Verification items for the finished model (mm, model axes). Coordinates: 2 decimals unless noted, no trailing zeros. Order: outer loops, then holes, each group sorted by start corner. A loop starts at its lowest first (then second) coordinate and runs counter-clockwise, first axis right, second up. Notation, with made-up numbers: M -30,34 L 2,34 A31 ccw 2,68 Z; hole C 8,65 d7. An arc over 180 degrees is marked long. Answer as a JSON object with one key per item and string values. Group by question number.
(1) Cross-section at B-B (y = 38). Enter the section's corners in (x, z).
(2) Cross-section at C-C (x = 34). Enter the section's corners in (y, z).
(3) Gauge pin test, flat ends, axial feed: pin 1 Ø0.9 at (y, z) = (62, 2) entering from -X; pin 2 Ø1.5 at (y, z) = (-0.5, 1) entering from -X; pin 3 Ø1.5 at (x, z) = (-69.5, 1) entering from +Y. Record the tip position at first contact, or that the pin passes through.
(4) Cross-section at A-A (x = 68.5). Enter the section's corners in (y, z), plus the area to 3 significant figures.
(5) Material ranges on line 1 (X direction, y = 43, z = 1.1); line 2 (X direction, y = 21.5, z = 1.95); line 3 (Y direction, x = 20.5, z = 1.6), recorded low to high.
(6) Cross-section at D-D (z = 1.65). Count the separate pieces of the cut face and the enclosed holes in it, plus the area to 3 significant figures.
from build123d import *

# Parameters (mm, degrees)
SKETCH1_R                     = 83.5
BOSS_EXTRUDE1_DEPTH           = 3
FACE_FLATTENING_REACH         = 120.125
SKETCH10_W                    = 98.960633138
SKETCH10_H                    = 16.23969765
SIDE_RIB_SLOT_DEPTH           = 10
RIB_TAB_CLEARANCE_SLOT_REACH  = 120.125
SKETCH5_W                     = 3.2
SKETCH5_H                     = 5
SKETCH5_H_2                   = 26
SIDE_RIB_SLOT_PATTERN_COUNT   = 2
EYE_PLATE_SLOTS_REACH         = 120.104
SKETCH3_R                     = 3
SKETCH3_W                     = 8.4
SKETCH3_H                     = 4.684444021
FACE_START                    = -3
FACE_PLATE_TABS_OUTLINE_W     = 2
FACE_PLATE_TABS_OUTLINE_H     = 4.476977338
FACE_PLATE_TABS_DEPTH         = 3
SKETCH11_W                    = 2
SKETCH11_H                    = 4.476977338
FACE_PLATE_TAB_RELIEF_DEPTH   = 3
ACTUATOR_CLEARANCE_SLOT_REACH = 120.104
SKETCH4_R                     = 4
EYE_PLATE_RELIEF_REACH        = 120.104


# Read off the part's stored shape, not the designer's step: face plate tabs
with BuildPart() as part:
    # Sketch1 → Boss-Extrude1 (new body)
    with BuildSketch(Plane.XY):
        Circle(SKETCH1_R)
    extrude(amount=BOSS_EXTRUDE1_DEPTH)

    # Sketch10 → face flattening (cut, up to next)
    with BuildSketch(Plane.XY.offset(3), mode=Mode.PRIVATE) as face_flattening_sk1:
        with Locations((0, 75.380151175)):
            Rectangle(SKETCH10_W, SKETCH10_H)
    face_flattening_tool1 = extrude(face_flattening_sk1.sketch, amount=-FACE_FLATTENING_REACH, mode=Mode.PRIVATE) & part.part
    add(face_flattening_tool1.solids().sort_by_distance((0, 75.380151, 3))[0], mode=Mode.SUBTRACT)

    # Sketch7 → side rib slot (cut)
    with BuildSketch(Plane.XY.offset(3)):
        with BuildLine():
            Line((-72.5, 1.635889894), (-72.5, 4.635889894))
            Line((-72.5, 4.635889894), (-66.5, 4.635889894))
            ThreePointArc((-66.5, 4.635889894), (-65.75, 5.385889894), (-66.5, 6.135889894))
            Line((-66.5, 6.135889894), (-87.5, 6.135889894))
            Line((-87.5, 6.135889894), (-87.5, -1.564110106))
            Line((-87.5, -1.564110106), (-72.5, -1.564110106))
            Line((-72.5, -1.564110106), (-59.391745722, -1.564110106))
            ThreePointArc((-59.391745722, -1.564110106), (-58.11423896, -2.394190801), (-57.5, -1))
            Line((-57.5, -1), (-57.5, 1))
            ThreePointArc((-57.5, 1), (-58.079561495, 2.383159214), (-59.379795897, 1.635889894))
            Line((-59.379795897, 1.635889894), (-70.5, 1.635889894))
            ThreePointArc((-70.5, 1.635889894), (-71.5, 1.035889894), (-72.5, 1.635889894))
        make_face()
    side_rib_slot = extrude(amount=-SIDE_RIB_SLOT_DEPTH, mode=Mode.SUBTRACT)

    # Sketch5 → rib tab clearance slot (cut, up to next)
    with BuildSketch(Plane.XY.offset(3), mode=Mode.PRIVATE) as rib_tab_clearance_slot_sk1:
        with Locations((0, 45)):
            Rectangle(SKETCH5_W, SKETCH5_H)
    rib_tab_clearance_slot_tool1 = extrude(rib_tab_clearance_slot_sk1.sketch, amount=-RIB_TAB_CLEARANCE_SLOT_REACH, mode=Mode.PRIVATE) & part.part
    # Sketch5 → rib tab clearance slot (cut, up to next)
    with BuildSketch(Plane.XY.offset(3), mode=Mode.PRIVATE) as rib_tab_clearance_slot_sk2:
        with Locations((0, 70.5)):
            Rectangle(SKETCH5_W, SKETCH5_H_2)
    rib_tab_clearance_slot_tool2 = extrude(rib_tab_clearance_slot_sk2.sketch, amount=-RIB_TAB_CLEARANCE_SLOT_REACH, mode=Mode.PRIVATE) & part.part
    # Sketch5 → rib tab clearance slot (cut, up to next)
    with BuildSketch(Plane.XY.offset(3), mode=Mode.PRIVATE) as rib_tab_clearance_slot_sk3:
        with Locations((0, -70.5)):
            Rectangle(SKETCH5_W, SKETCH5_H_2)
    rib_tab_clearance_slot_tool3 = extrude(rib_tab_clearance_slot_sk3.sketch, amount=-RIB_TAB_CLEARANCE_SLOT_REACH, mode=Mode.PRIVATE) & part.part
    # Sketch5 → rib tab clearance slot (cut, up to next)
    with BuildSketch(Plane.XY.offset(3), mode=Mode.PRIVATE) as rib_tab_clearance_slot_sk4:
        with Locations((0, -45)):
            Rectangle(SKETCH5_W, SKETCH5_H)
    rib_tab_clearance_slot_tool4 = extrude(rib_tab_clearance_slot_sk4.sketch, amount=-RIB_TAB_CLEARANCE_SLOT_REACH, mode=Mode.PRIVATE) & part.part
    add(rib_tab_clearance_slot_tool1.solids().sort_by_distance((0, 45, 3))[0], mode=Mode.SUBTRACT)
    add(rib_tab_clearance_slot_tool2.solids().sort_by_distance((0, 70.5, 3))[0], mode=Mode.SUBTRACT)
    add(rib_tab_clearance_slot_tool3.solids().sort_by_distance((0, -70.5, 3))[0], mode=Mode.SUBTRACT)
    add(rib_tab_clearance_slot_tool4.solids().sort_by_distance((0, -45, 3))[0], mode=Mode.SUBTRACT)

    # side rib slot pattern: side rib slot ×2 about axis
    side_rib_slot_pattern_axis = Axis((0, 0, 0), (0, 0, 1))
    for i in range(1, SIDE_RIB_SLOT_PATTERN_COUNT):
        add(side_rib_slot.rotate(side_rib_slot_pattern_axis, i * 360 / SIDE_RIB_SLOT_PATTERN_COUNT), mode=Mode.SUBTRACT)

    # Sketch3 → eye plate slots (cut, up to next)
    with BuildSketch(Plane.XY.offset(3), mode=Mode.PRIVATE) as eye_plate_slots_sk1:
        with Locations((-25, 20)):
            Circle(SKETCH3_R)
    eye_plate_slots_tool1 = extrude(eye_plate_slots_sk1.sketch, amount=-EYE_PLATE_SLOTS_REACH, mode=Mode.PRIVATE) & part.part
    # Sketch3 → eye plate slots (cut, up to next)
    with BuildSketch(Plane.XY.offset(3), mode=Mode.PRIVATE) as eye_plate_slots_sk2:
        with Locations((25, 20)):
            Circle(SKETCH3_R)
    eye_plate_slots_tool2 = extrude(eye_plate_slots_sk2.sketch, amount=-EYE_PLATE_SLOTS_REACH, mode=Mode.PRIVATE) & part.part
    # Sketch3 → eye plate slots (cut, up to next)
    with BuildSketch(Plane.XY.offset(3), mode=Mode.PRIVATE) as eye_plate_slots_sk3:
        with Locations((-51, 44.926435594)):
            Rectangle(SKETCH3_W, SKETCH3_H)
    eye_plate_slots_tool3 = extrude(eye_plate_slots_sk3.sketch, amount=-EYE_PLATE_SLOTS_REACH, mode=Mode.PRIVATE) & part.part
    # Sketch3 → eye plate slots (cut, up to next)
    with BuildSketch(Plane.XY.offset(3), mode=Mode.PRIVATE) as eye_plate_slots_sk4:
        with Locations((51, 44.926435594)):
            Rectangle(SKETCH3_W, SKETCH3_H)
    eye_plate_slots_tool4 = extrude(eye_plate_slots_sk4.sketch, amount=-EYE_PLATE_SLOTS_REACH, mode=Mode.PRIVATE) & part.part
    add(eye_plate_slots_tool1.solids().sort_by_distance((-25, 20, 3))[0], mode=Mode.SUBTRACT)
    add(eye_plate_slots_tool2.solids().sort_by_distance((25, 20, 3))[0], mode=Mode.SUBTRACT)
    add(eye_plate_slots_tool3.solids().sort_by_distance((-51, 44.926436, 3))[0], mode=Mode.SUBTRACT)
    add(eye_plate_slots_tool4.solids().sort_by_distance((51, 44.926436, 3))[0], mode=Mode.SUBTRACT)

    # face plate tabs outline → face plate tabs (add)
    with BuildSketch(Plane.XY.offset(3).offset(FACE_START)):
        Polygon((24.9, 67.26030235), (24.9, 77.837279688), (19.9, 77.837279688), (19.4, 74.837279688), (19.9, 74.837279688), (19.9, 71.737279688), (17.9, 71.737279688), (17.9, 67.26030235), align=None)
        with Locations((32.9, 69.498791019)):
            Rectangle(FACE_PLATE_TABS_OUTLINE_W, FACE_PLATE_TABS_OUTLINE_H)
        Polygon((26.9, 77.837279688), (26.9, 67.26030235), (29.9, 67.26030235), (29.9, 71.737279688), (30.1, 74.837279688), (30.6, 74.837279688), (30.1, 77.837279688), align=None)
        Polygon((-25.1, 67.26030235), (-25.1, 77.837279688), (-30.1, 77.837279688), (-30.6, 74.837279688), (-30.1, 74.837279688), (-30.1, 71.737279688), (-32.1, 71.737279688), (-32.1, 67.26030235), align=None)
        with Locations((-17.1, 69.498791019)):
            Rectangle(FACE_PLATE_TABS_OUTLINE_W, FACE_PLATE_TABS_OUTLINE_H)
        Polygon((-23.1, 77.837279688), (-23.1, 67.26030235), (-20.1, 67.26030235), (-20.1, 71.737279688), (-19.9, 74.837279688), (-19.4, 74.837279688), (-19.9, 77.837279688), align=None)
    extrude(amount=FACE_PLATE_TABS_DEPTH)

    # Sketch11 → face plate tab relief (cut)
    with BuildSketch(Plane.XY.offset(3).offset(FACE_START)):
        with BuildLine():
            Line((29.9, 66.837279688), (29.9, 67.26030235))
            Line((29.9, 67.26030235), (31.9, 71.737279688))
            Line((31.9, 71.737279688), (33.9, 71.737279688))
            Line((33.9, 71.737279688), (33.9, 67.26030235))
            Line((33.9, 67.26030235), (31.9, 67.26030235))
            Line((31.9, 67.26030235), (31.9, 66.837279688))
            ThreePointArc((31.9, 66.837279688), (30.9, 65.837279688), (29.9, 66.837279688))
        make_face()
        with BuildLine():
            Line((24.9, 66.837279688), (24.9, 67.26030235))
            Line((24.9, 67.26030235), (26.9, 67.26030235))
            Line((26.9, 67.26030235), (26.9, 66.837279688))
            ThreePointArc((26.9, 66.837279688), (25.9, 65.837279688), (24.9, 66.837279688))
        make_face()
        with Locations((18.9, 69.498791019)):
            Rectangle(SKETCH11_W, SKETCH11_H)
        with BuildLine():
            Line((-25.1, 66.837279688), (-25.1, 67.26030235))
            Line((-25.1, 67.26030235), (-23.1, 67.26030235))
            Line((-23.1, 67.26030235), (-23.1, 66.837279688))
            ThreePointArc((-23.1, 66.837279688), (-24.1, 65.837279688), (-25.1, 66.837279688))
        make_face()
        with BuildLine():
            Line((-20.1, 66.837279688), (-20.1, 67.26030235))
            Line((-20.1, 67.26030235), (-18.1, 71.737279688))
            Line((-18.1, 71.737279688), (-16.1, 71.737279688))
            Line((-16.1, 71.737279688), (-16.1, 67.26030235))
            Line((-16.1, 67.26030235), (-18.1, 67.26030235))
            Line((-18.1, 67.26030235), (-18.1, 66.837279688))
            ThreePointArc((-18.1, 66.837279688), (-19.1, 65.837279688), (-20.1, 66.837279688))
        make_face()
        with Locations((-31.1, 69.498791019)):
            Rectangle(SKETCH11_W, SKETCH11_H)
    extrude(amount=FACE_PLATE_TAB_RELIEF_DEPTH, mode=Mode.SUBTRACT)

    # Sketch4 → actuator clearance slot (cut, up to next)
    with BuildSketch(Plane.XY.offset(3), mode=Mode.PRIVATE) as actuator_clearance_slot_sk1:
        with Locations((19.684125428, -34.734157019)):
            Circle(SKETCH4_R)
    actuator_clearance_slot_tool1 = extrude(actuator_clearance_slot_sk1.sketch, amount=-ACTUATOR_CLEARANCE_SLOT_REACH, mode=Mode.PRIVATE) & part.part
    # Sketch4 → actuator clearance slot (cut, up to next)
    with BuildSketch(Plane.XY.offset(3), mode=Mode.PRIVATE) as actuator_clearance_slot_sk2:
        with BuildLine():
            Line((-6, 23.963301095), (-6, -43.311948564))
            ThreePointArc((-6, -43.311948564), (-12, -49.311948564), (-18, -43.311948564))
            Line((-18, -43.311948564), (-18, 23.963301095))
            ThreePointArc((-18, 23.963301095), (-12, 29.963301095), (-6, 23.963301095))
        make_face()
    actuator_clearance_slot_tool2 = extrude(actuator_clearance_slot_sk2.sketch, amount=-ACTUATOR_CLEARANCE_SLOT_REACH, mode=Mode.PRIVATE) & part.part
    add(actuator_clearance_slot_tool1.solids().sort_by_distance((19.684125, -34.734157, 3))[0], mode=Mode.SUBTRACT)
    add(actuator_clearance_slot_tool2.solids().sort_by_distance((-12, -9.674324, 3))[0], mode=Mode.SUBTRACT)

    # Sketch12 → eye plate relief (cut, up to next)
    with BuildSketch(Plane.XY.offset(3), mode=Mode.PRIVATE) as eye_plate_relief_sk1:
        with BuildLine():
            Line((54.501230688, 63.26030235), (48.480316569, 63.26030235))
            ThreePointArc((48.480316569, 63.26030235), (45.651889444, 64.431875226), (44.480316569, 67.26030235))
            Line((44.480316569, 67.26030235), (54.501230688, 67.26030235))
            Line((54.501230688, 67.26030235), (54.501230688, 63.26030235))
        make_face()
    eye_plate_relief_tool1 = extrude(eye_plate_relief_sk1.sketch, amount=-EYE_PLATE_RELIEF_REACH, mode=Mode.PRIVATE) & part.part
    # Sketch12 → eye plate relief (cut, up to next)
    with BuildSketch(Plane.XY.offset(3), mode=Mode.PRIVATE) as eye_plate_relief_sk2:
        with BuildLine():
            Line((-54.501230688, 67.26030235), (-44.480316569, 67.26030235))
            ThreePointArc((-44.480316569, 67.26030235), (-45.651889444, 64.431875226), (-48.480316569, 63.26030235))
            Line((-48.480316569, 63.26030235), (-54.501230688, 63.26030235))
            Line((-54.501230688, 63.26030235), (-54.501230688, 67.26030235))
        make_face()
    eye_plate_relief_tool2 = extrude(eye_plate_relief_sk2.sketch, amount=-EYE_PLATE_RELIEF_REACH, mode=Mode.PRIVATE) & part.part
    add(eye_plate_relief_tool1.solids().sort_by_distance((49.876481, 65.36397, 3))[0], mode=Mode.SUBTRACT)
    add(eye_plate_relief_tool2.solids().sort_by_distance((-49.876481, 65.36397, 3))[0], mode=Mode.SUBTRACT)


solid = part.part
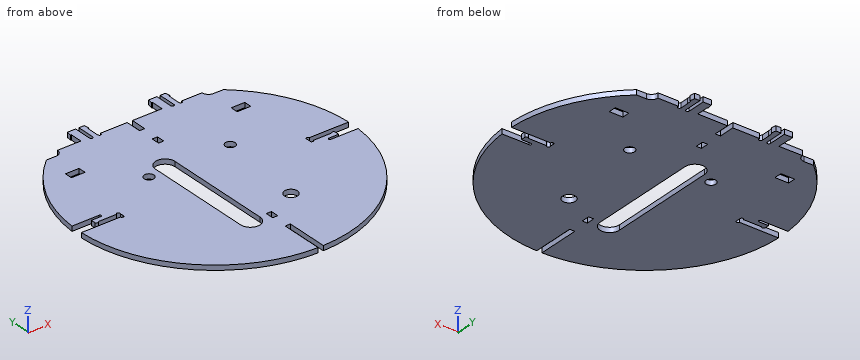
Taken from the geometry:
{
 "1": {"outline": "M -74.35,0 L 74.35,0 L 74.35,3 L -74.35,3 Z"},
 "2": {"outline": "M -76.26,0 L 67.26,0 L 67.26,3 L -76.26,3 Z"},
 "3": {"pin 1": "stops at x = -56.43", "pin 2": "stops at x = -57.5", "pin 3": "stops at y = 47.39"},
 "4": {"outline": "M -47.75,0 L -6.14,0 L -6.14,3 L -47.75,3 Z; M -4.64,0 L -1.64,0 L -1.64,3 L -4.64,3 Z; M 1.56,0 L 47.75,0 L 47.75,3 L 1.56,3 Z", "area": "272 mm²"},
 "5": {"line 1": "x = -71.58 to -55.2, -46.8 to -1.6, 1.6 to 46.8, 55.2 to 71.58", "line 2": "x = -80.68 to -27.6, -22.4 to -18, -6 to 22.4, 27.6 to 80.68", "line 3": "y = -80.94 to -38.65, -30.82 to 77.84"},
 "6": {"separate pieces": "1", "enclosed holes": "8", "area": "19,400 mm²"}
}
